Here's how the part is built. I have some questions about the finished solid (model axes, mm). Round coordinates to 2 decimals unless told otherwise and drop trailing zeros. Loops run counter-clockwise (first coordinate to the right, second up) from the corner with the lowest first, then second, coordinate; pieces in that order, holes last. Notation, with made-up numbers: M -38.75,-27 L -1.75,-27 A28 ccw -1.75,7 Z; hole C 5.5,6 d2. An arc over 180 degrees is marked long. Answer as a JSON object with one key per item and string values.
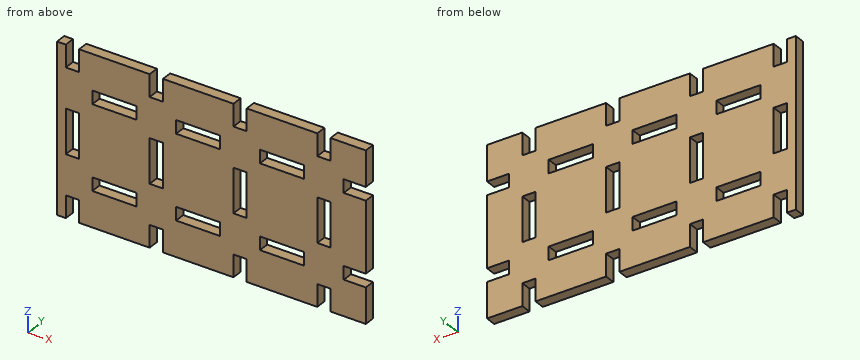
from build123d import *

# Parameters (mm, degrees)
ESQUISSE1_W             = 175
ESQUISSE1_H             = 95
BOSS_EXTRU_1_DEPTH      = 6
ESQUISSE9_W             = 25
ESQUISSE9_H             = 7.5
ESQUISSE9_W_2           = 12.5
ESQUISSE9_W_3           = 7.5
ESQUISSE9_H_2           = 12.5
ESQUISSE9_H_3           = 25
ENL_V_MAT_EXTRU_1_DEPTH = 6000


with BuildPart() as part:
    # Esquisse1 → Boss.-Extru.1 (new body)
    with BuildSketch(Plane(origin=(0, 0, 0), x_dir=(1, 0, 0), z_dir=(0, 1, 0))):
        with Locations((-87.5, -47.5)):
            Rectangle(ESQUISSE1_W, ESQUISSE1_H)
    extrude(amount=BOSS_EXTRU_1_DEPTH)

    # Esquisse9 → Enlèv. mat.-Extru.1 (cut)
    with BuildSketch(Plane(origin=(0, 6, 0), x_dir=(1, 0, 0), z_dir=(0, 1, 0))):
        with Locations((-142.5, -23.75)):
            Rectangle(ESQUISSE9_W, ESQUISSE9_H)
        with Locations((-142.5, -71.25)):
            Rectangle(ESQUISSE9_W, ESQUISSE9_H)
        with Locations((-95, -71.25)):
            Rectangle(ESQUISSE9_W, ESQUISSE9_H)
        with Locations((-95, -23.75)):
            Rectangle(ESQUISSE9_W, ESQUISSE9_H)
        with Locations((-47.5, -23.75)):
            Rectangle(ESQUISSE9_W, ESQUISSE9_H)
        with Locations((-6.25, -23.75)):
            Rectangle(ESQUISSE9_W_2, ESQUISSE9_H)
        with Locations((-47.5, -71.25)):
            Rectangle(ESQUISSE9_W, ESQUISSE9_H)
        with Locations((-6.25, -71.25)):
            Rectangle(ESQUISSE9_W_2, ESQUISSE9_H)
        with Locations((-166.25, -88.75)):
            Rectangle(ESQUISSE9_W_3, ESQUISSE9_H_2)
        with Locations((-166.25, -47.5)):
            Rectangle(ESQUISSE9_W_3, ESQUISSE9_H_3)
        with Locations((-166.25, -6.25)):
            Rectangle(ESQUISSE9_W_3, ESQUISSE9_H_2)
        with Locations((-118.75, -88.75)):
            Rectangle(ESQUISSE9_W_3, ESQUISSE9_H_2)
        with Locations((-71.25, -88.75)):
            Rectangle(ESQUISSE9_W_3, ESQUISSE9_H_2)
        with Locations((-23.75, -88.75)):
            Rectangle(ESQUISSE9_W_3, ESQUISSE9_H_2)
        with Locations((-118.75, -47.5)):
            Rectangle(ESQUISSE9_W_3, ESQUISSE9_H_3)
        with Locations((-71.25, -47.5)):
            Rectangle(ESQUISSE9_W_3, ESQUISSE9_H_3)
        with Locations((-23.75, -47.5)):
            Rectangle(ESQUISSE9_W_3, ESQUISSE9_H_3)
        with Locations((-118.75, -6.25)):
            Rectangle(ESQUISSE9_W_3, ESQUISSE9_H_2)
        with Locations((-71.25, -6.25)):
            Rectangle(ESQUISSE9_W_3, ESQUISSE9_H_2)
        with Locations((-23.75, -6.25)):
            Rectangle(ESQUISSE9_W_3, ESQUISSE9_H_2)
    extrude(amount=-ENL_V_MAT_EXTRU_1_DEPTH, mode=Mode.SUBTRACT)


solid = part.part
Item 1: I want a section at C-C on x = -117.5. List the corners of the cut face in (y, z) for me, plus the area to 3 significant figures.
Solution:
{"outline": "M 0,12.5 L 6,12.5 L 6,35 L 0,35 Z; M 0,60 L 6,60 L 6,82.5 L 0,82.5 Z", "area": "270 mm2"}
Item 2: For P1, Ø1, axis at x = -110.5, y = 2.5, coming from the -Z side; P2, Ø3, axis at x = -24, y = 3.5, coming from the -Z side, each with a flat end and sliding along its axis, tell me the tip position at first contact or that it passes through.
Solution:
{"P1": "stops at z = 0", "P2": "stops at z = 12.5"}
Item 3: If I drill on L1, parallel to X at y = 4.8, z = 90.5; L2, parallel to Z at x = -154.5, y = 2.45; L3, parallel to Z at x = -117, y = 3.4, over which ranges is the centre line in solid material (lowest first)? Write a range as from..to.
Solution:
{"L1": "x = -175..-170, -162.5..-122.5, -115..-75, -67.5..-27.5, -20..0", "L2": "z = 0..20, 27.5..67.5, 75..95", "L3": "z = 12.5..35, 60..82.5"}
Item 4: I want a section at D-D on z = 9. List the corners of the cut face in (x, y) for me.
Solution:
{"outline": "M -175,0 L -170,0 L -170,6 L -175,6 Z; M -162.5,0 L -122.5,0 L -122.5,6 L -162.5,6 Z; M -115,0 L -75,0 L -75,6 L -115,6 Z; M -67.5,0 L -27.5,0 L -27.5,6 L -67.5,6 Z; M -20,0 L 0,0 L 0,6 L -20,6 Z"}
Item 5: I want a section at A-A on z = 70. List the corners of the cut face in (x, y) for me, plus the area to 3 significant figures.
Solution:
{"outline": "M -175,0 L -155,0 L -155,6 L -175,6 Z; M -130,0 L -107.5,0 L -107.5,6 L -130,6 Z; M -82.5,0 L -60,0 L -60,6 L -82.5,6 Z; M -35,0 L -12.5,0 L -12.5,6 L -35,6 Z", "area": "525 mm2"}
Item 6: I want a section at B-B on x = -40. List the corners of the cut face in (y, z) for me.
Solution:
{"outline": "M 0,0 L 6,0 L 6,20 L 0,20 Z; M 0,27.5 L 6,27.5 L 6,67.5 L 0,67.5 Z; M 0,75 L 6,75 L 6,95 L 0,95 Z"}
